Can you work these out from the model? Positions are in its coordinate system, mm. Give positions to 0.01 mm unless a question says otherwise; leave off trailing zeros. Loops run counter-clockwise (first coordinate to the right, second up) from the corner with the lowest first, then second, coordinate; pieces in that order, holes last. Notation, with made-up numbers: (20.5, 59) - (27.5, 59) arc R8 cw to (27.5, 66) - close; hole circle Ø10 at (69.5, 11). An arc over 180 degrees is marked (long way). Answer in a Markdown table with one row per item.
from build123d import *

# Parameters (mm, degrees)
TOPSKETCH1_R                        = 1.59
TOPBOSS_EXTRUDE1_DEPTH              = 2
FILLET1_R                           = 10
LINEARRAILHEIGHTSKETCH2_W           = 227.746666667
LINEARRAILHEIGHTSKETCH2_H           = 7
LINEARRAILHEIGHTBOSS_EXTRUDE2_DEPTH = 12
LINEARRAILHOLESSKETCH3_R            = 1.75
LINEARRAILHOLESCUT_EXTRUDE1_DEPTH   = 208.226612432
CONNECTINGPLATESKETCH1_W            = 25
CONNECTINGPLATESKETCH1_H            = 14
CONNECTINGPLATECUT_EXTRUDE1_DEPTH   = 4
FILLET2_R                           = 3.175


with BuildPart() as part:
    # TopSketch1 → TopBoss-Extrude1 (new body)
    with BuildSketch(Plane(origin=(0, 0, 0), x_dir=(1, 0, 0), z_dir=(0, 1, 0))):
        Polygon((0, 0), (34, 0), (34, 37.5), (0, 37.5), (0, 19.25), (-205.08, 19.25), (-205.08, 11.25), (0, 11.25), align=None)
        with Locations(Location((8.5, 32.5, 0), (0, 0, 270))):
            Circle(TOPSKETCH1_R, mode=Mode.SUBTRACT)
        with Locations(Location((8.5, 5, 0), (0, 0, 270))):
            Circle(TOPSKETCH1_R, mode=Mode.SUBTRACT)
        with Locations(Location((25.5, 18.75, 0), (0, 0, 270))):
            Circle(TOPSKETCH1_R, mode=Mode.SUBTRACT)
    extrude(amount=TOPBOSS_EXTRUDE1_DEPTH)

    # Fillet1
    fillet1_edges = [part.edges().sort_by_distance(p)[0] for p in [
        (0, 1, -37.5),
        (0, 1, 0),
    ]]
    fillet(fillet1_edges, radius=FILLET1_R)

    # LinearRailHEightSketch2 → LinearRailHeightBoss-Extrude2 (add)
    with BuildSketch(Plane(origin=(0, 2, 0), x_dir=(1, 0, 0), z_dir=(0, 1, 0))):
        with Locations((-91.206666667, 14.75)):
            Rectangle(LINEARRAILHEIGHTSKETCH2_W, LINEARRAILHEIGHTSKETCH2_H)
    extrude(amount=LINEARRAILHEIGHTBOSS_EXTRUDE2_DEPTH)

    # LinearRailHolesSketch3 → LinearRailHolesCut-Extrude1 (cut, through all)
    with BuildSketch(Plane.XY.offset(-11.25)):
        with Locations((-192.58, 8)):
            Circle(LINEARRAILHOLESSKETCH3_R)
        with Locations((-167.58, 8)):
            Circle(LINEARRAILHOLESSKETCH3_R)
        with Locations((-142.58, 8)):
            Circle(LINEARRAILHOLESSKETCH3_R)
        with Locations((-117.58, 8)):
            Circle(LINEARRAILHOLESSKETCH3_R)
        with Locations((-92.58, 8)):
            Circle(LINEARRAILHOLESSKETCH3_R)
        with Locations((-67.58, 8)):
            Circle(LINEARRAILHOLESSKETCH3_R)
        with Locations((-42.58, 8)):
            Circle(LINEARRAILHOLESSKETCH3_R)
        with Locations((-17.58, 8)):
            Circle(LINEARRAILHOLESSKETCH3_R)
    extrude(amount=-LINEARRAILHOLESCUT_EXTRUDE1_DEPTH, mode=Mode.SUBTRACT)

    # ConnectingPlateSketch1 → ConnectingPlateCut-Extrude1 (cut)
    with BuildSketch(Plane.XY.offset(-11.25)):
        with Locations((-192.58, 7)):
            Rectangle(CONNECTINGPLATESKETCH1_W, CONNECTINGPLATESKETCH1_H)
    extrude(amount=-CONNECTINGPLATECUT_EXTRUDE1_DEPTH, mode=Mode.SUBTRACT)

    # Fillet2
    fillet2_edges = [part.edges().sort_by_distance(p)[0] for p in [
        (22.666666667, 14, -14.75),
    ]]
    fillet(fillet2_edges, radius=FILLET2_R)


solid = part.part
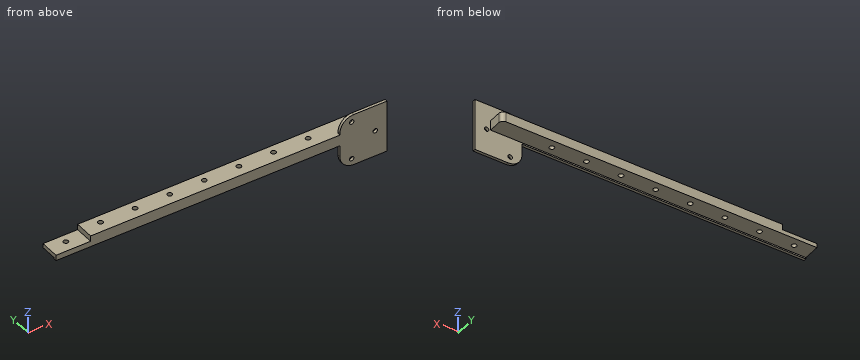
Q1. Imagine slicing it at B-B, the plane y = 4.25. Write out the boundary of the cut face in (x, z).
Checked values:
| item | result |
|---|---|
| outline | (-205.08, -18.25) - (22.67, -18.25) - (22.67, -11.25) - (-180.08, -11.25) - (-180.08, -15.25) - (-205.08, -15.25) - close |
Q2. Imagine slicing it at A-A, the plane x = -112. Write out the boundary of the cut face in (y, z).
Checked values:
| item | result |
|---|---|
| outline | (0, -19.25) - (2, -19.25) - (2, -18.25) - (14, -18.25) - (14, -11.25) - (0, -11.25) - close |
Q3. If I drill on line 1 (X direction, y = 0.8, z = -18.75); line 2 (Z direction, x = -72, y = 8.75); line 3 (Y direction, x = -142.58, z = -16), over which ranges is the centre line in solid material (lowest first)? Write a range as [from, to].
Checked values:
| item | result |
|---|---|
| line 1 | x = [-205.08, 23.91], [27.09, 34] |
| line 2 | z = [-18.25, -11.25] |
| line 3 | y = [0, 6.25], [9.75, 14] |
Q4. For pin 1 (2 mm diameter, centred on x = -42.58, y = 8, fed in from -Z); pin 2 (2 mm diameter, centred on x = -55.5, y = 1, fed in from -Z); pin 3 (3 mm diameter, centred on x = -71.5, y = 2, fed in from +Z); pin 4 (4 mm diameter, centred on x = -37.5, y = 10, fed in from -Z), each with a flat end and sliding along its axis, tell me the tip position at first contact or that it passes through.
Checked values:
| item | result |
|---|---|
| pin 1 | passes through |
| pin 2 | stops at z = -19.25 |
| pin 3 | stops at z = -11.25 |
| pin 4 | stops at z = -18.25 |
